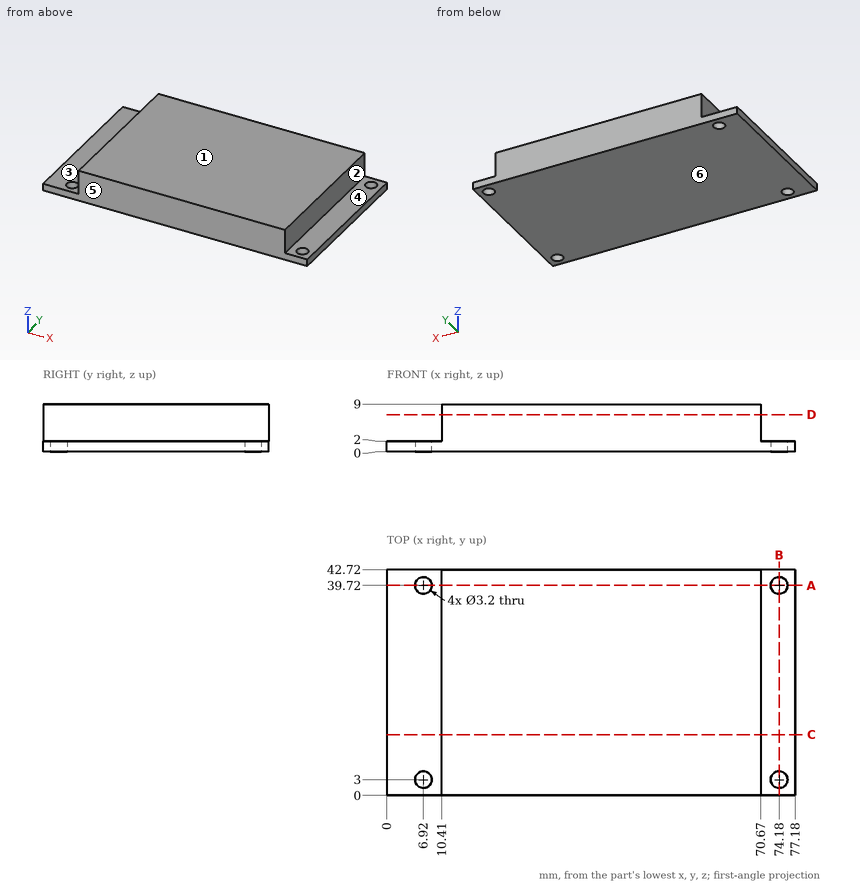
Could you check a few things on this drawing? It's one solid part, dimensions in mm from its lowest x, y, z. A direction names the side the tool comes from. Give positions to 0.01 mm unless a question says otherwise; leave off trailing zeros. Order: outer loops, then holes, each group sorted by start corner. A loop starts at its lowest first (then second) coordinate and runs counter-clockwise, first axis right, second up. Notation, with made-up numbers: (-29, -14.5) - (21, -14.5) arc R18 ccw to (21, -10.5) - close; hole circle Ø3 at (31.5, -5). An arc over 180 degrees is marked (long way). One line per question, with ' | ' between items. Start each with the question number.
Item 1: I want a section at A-A on y = 39.72. Write out the boundary of the cut face in (x, z).
Item 2: I'm going to push flat-ended pins straight in: pin 1 Ø2 at (y, z) = (6, 6.5) entering from +X; pin 2 Ø5 at (x, y) = (74.18, 3) entering from +Z; pin 3 Ø2.5 at (x, y) = (6.92, 39.72) entering from +Z. Where does each tip first touch, or does it pass through?
Item 3: I want a section at B-B on x = 74.18. Write out the boundary of the cut face in (y, z).
Item 4: I want a section at C-C on y = 11.5. Write out the boundary of the cut face in (x, z).
Item 5: I want a section at D-D on z = 7. Write out the boundary of the cut face in (x, y).
Item 6: I need wall thicknesses on probe 1 along Y at (x, z) = (6.92, 0.9); probe 2 along X at (y, z) = (3, 1.3); probe 3 along X at (y, z) = (41, 1). Which ranges of each line are inside material? Lowest first, please. Write a range as [from, to].
Item 7: For the marked faces 1, 2 and 3, which set-ups out of +Z, -Z, +X, -X, +Y, -Y let a thin tool reach every point of the face, with its end or its side?
Item 8: Thinking about a two-plate mould opening in Z: for the marked faces 4, 5 and 6, which applies, pulls with the +Z half, pulls with the -Z half, needs draft (parallel to the pull), parting line crosses it, or undercut?
Verdict:
1) outline: (0, 0) - (5.32, 0) - (5.32, 2) - (0, 2) - close; (8.52, 0) - (72.58, 0) - (72.58, 2) - (70.67, 2) - (70.67, 9) - (10.41, 9) - (10.41, 2) - (8.52, 2) - close; (75.78, 0) - (77.18, 0) - (77.18, 2) - (75.78, 2) - close
2) pin 1: x = 70.67 | pin 2: z = 2 | pin 3: through
3) outline: (0, 0) - (1.4, 0) - (1.4, 2) - (0, 2) - close; (4.6, 0) - (38.12, 0) - (38.12, 2) - (4.6, 2) - close; (41.32, 0) - (42.72, 0) - (42.72, 2) - (41.32, 2) - close
4) outline: (0, 0) - (77.18, 0) - (77.18, 2) - (70.67, 2) - (70.67, 9) - (10.41, 9) - (10.41, 2) - (0, 2) - close
5) outline: (10.41, 0) - (70.67, 0) - (70.67, 42.72) - (10.41, 42.72) - close
6) probe 1: [0, 1.4], [4.6, 38.12], [41.32, 42.72] | probe 2: [0, 5.32], [8.52, 72.58], [75.78, 77.18] | probe 3: [0, 5.96], [7.88, 73.22], [75.14, 77.18]
7) face 1: +Z, +X, -X, +Y, -Y | face 2: +Z, +X, +Y, -Y | face 3: +Z, -X, +Y, -Y
8) face 4: pulls with the +Z half | face 5: needs draft | face 6: pulls with the -Z half
